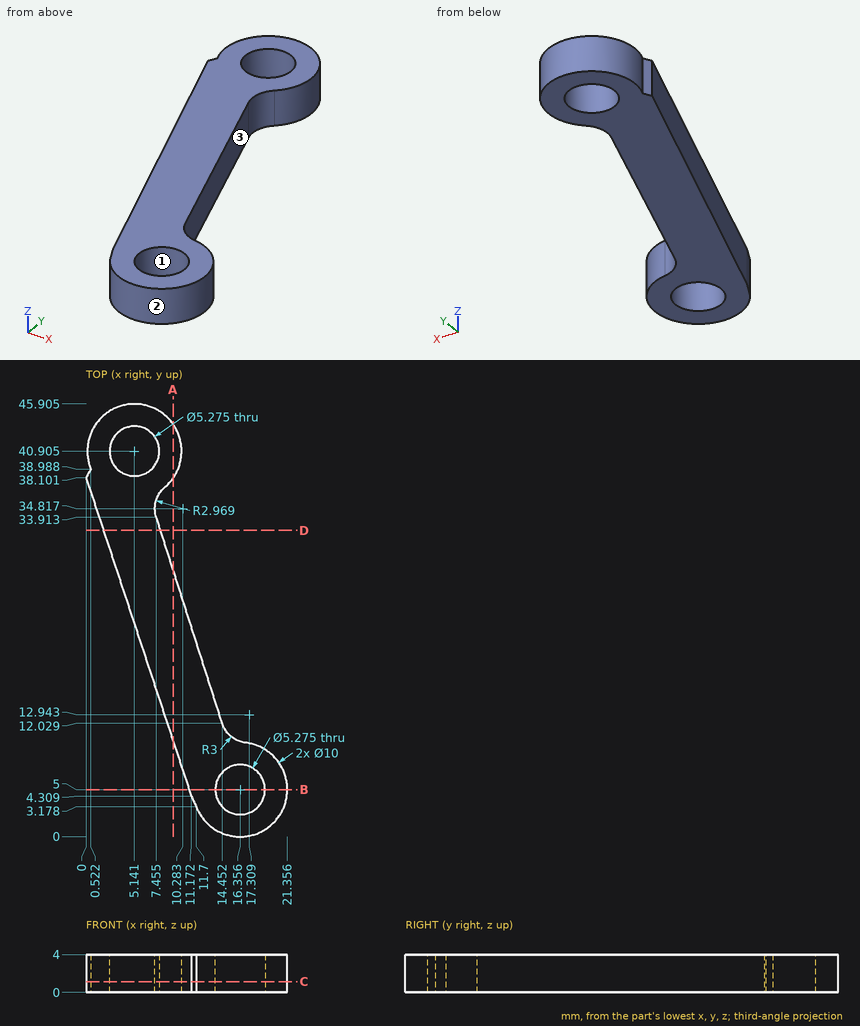
Print and shaded views of the part. All mm, measured from the part's lowest x, y and z. Give positions to 0.01 mm unless a question says otherwise; leave off trailing zeros. Loops run counter-clockwise (first coordinate to the right, second up) from the corner with the lowest first, then second, coordinate; pieces in that order, holes last.
1) Flat gauge pins, fed straight in: pin 1 Ø3 at (x, y) = (10, 36) entering from +Z; pin 2 Ø7 at (x, y) = (5.14, 40.9) entering from -Z; pin 3 Ø1 at (x, z) = (8.5, 0.5) entering from +Y (1 decimal); pin 4 Ø1 at (y, z) = (12.5, 2.5) entering from +X. Where does each tip first touch, or does it go through?
2) Pull direction X, two halves, no side cores. Call the marked faces 1, 2 and 3: +X half, -X half, draft (parallel to the pull), parting line (faces both ways), or undercut.
3) Wall check: line 1 (Y direction, x = 17.25, z = 2.8); line 2 (Y direction, x = 14.75, z = 0.35) (1 decimal); line 3 (Y direction, x = 20.25, z = 3.1) (1 decimal). Give the ranges that are in metal, low to high.
4) Saw through at A-A (x = 9.25). Write the cut outline in (y, z).
5) Saw through at D-D (y = 32.5). Write the cut outline in (x, z).
6) Saw through at C-C (z = 1.15). Write the cut outline in (x, y) (1 decimal), plus the area to 3 significant figures.
7) Saw through at B-B (y = 5). Write the cut outline in (x, z) (1 decimal).
Answer block:
1. pin 1: passes through
1. pin 2: stops at z = 0
1. pin 3: stops at y = 45
1. pin 4: stops at x = 14.46
2. face 1: undercut
2. face 2: parting line
2. face 3: +X half
3. line 1: y = 0.08 to 2.52, 7.48 to 9.92
3. line 2: y = 0.3 to 2.9, 7.1 to 11.4
3. line 3: y = 1.9 to 8.1
4. outline: (10.12, 0) - (28.3, 0) - (28.3, 4) - (10.12, 4) - close; (38.06, 0) - (43.75, 0) - (43.75, 4) - (38.06, 4) - close
5. outline: (1.85, 0) - (7.91, 0) - (7.91, 4) - (1.85, 4) - close
6. outline: (0, 38.1) - (11.2, 4.3) - (11.7, 3.2) arc R5 ccw (long way) to (17, 10) arc R3 cw to (14.5, 12) - (7.5, 33.9) arc R3 cw to (8.4, 37.1) arc R5 ccw (long way) to (0.5, 39) - close; hole circle Ø5.3 at (5.1, 40.9); hole circle Ø5.3 at (16.4, 5)
6. area: 286 mm2
7. outline: (10.9, 0) - (13.7, 0) - (13.7, 4) - (10.9, 4) - close; (19, 0) - (21.4, 0) - (21.4, 4) - (19, 4) - close
